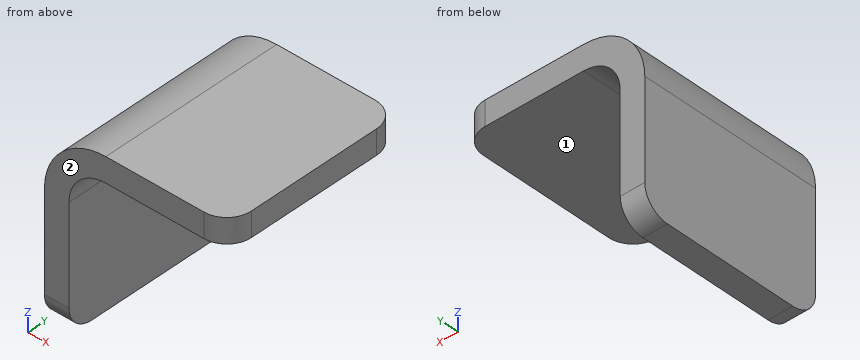
from build123d import *

# Parameters (mm, degrees)
F1_DEPTH = 15
F2_R     = 3
F3_R     = 5
F4_R     = 2


with BuildPart() as f1:
    # F0 (on Front) → F1 (new body)
    with BuildSketch(Plane.XZ):
        Polygon((15, 0), (0, 0), (0, -15), (2, -15), (2, -2), (15, -2), align=None)
    extrude(amount=F1_DEPTH)

    # F2
    f2_edges = [f1.edges().sort_by_distance(p)[0] for p in [
        (2, -7.5, -2),
    ]]
    fillet(f2_edges, radius=F2_R)

    # F3
    f3_edges = [f1.edges().sort_by_distance(p)[0] for p in [
        (0, -7.5, 0),
    ]]
    fillet(f3_edges, radius=F3_R)

    # F4
    f4_edges = [f1.edges().sort_by_distance(p)[0] for p in [
        (15, -15, -1),
        (15, 0, -1),
        (1, -15, -15),
        (1, 0, -15),
    ]]
    fillet(f4_edges, radius=F4_R)


solid = f1.part
For this review, take the finished solid that the model builds, in its own axes (mm). Face numbers are marked on the shaded views. A direction names the side the tool comes from. Round coordinates to 2 decimals unless told otherwise and drop trailing zeros. Order: outer loops, then holes, each group sorted by start corner. A loop starts at its lowest first (then second) coordinate and runs counter-clockwise, first axis right, second up. Notation, with made-up numbers: (6.5, -38) -> (10.5, -38) arc R24 ccw to (10.5, -14) -> close; hole circle Ø3 at (-5.5, -27.5). An arc over 180 degrees is marked (long way). Put each result on its own line as item: value.
Q1. Machinability: for the marked faces 1 and 2, which of the approach directions +Z, -Z, +X, -X, +Y, -Y give a long, thin tool a straight path to every point of the face, cutting with its end or side? Answer none if there is none.
Check result:
face 1: -Z, +X, +Y, -Y
face 2: +Z, -Z, +X, -X, -Y
Q2. Add section C-C on x = 11.5. Write out the cut boundary in (y, z).
Check result:
outline: (-15, -2) -> (0, -2) -> (0, 0) -> (-15, 0) -> close
Q3. For probe 1 along X at (y, z) = (-9.5, -12.75); probe 2 along Z at (x, y) = (8.5, -7.25); probe 3 along Z at (x, y) = (1, -8.75), list the stretches that pass through material, from the lowest coordinate up. Write a range as [from, to].
Check result:
probe 1: [0, 2]
probe 2: [-2, 0]
probe 3: [-15, -2]
Q4. Add section D-D on z = -1. Write out the cut boundary in (x, y).
Check result:
outline: (2, -15) -> (13, -15) arc R2 ccw to (15, -13) -> (15, -2) arc R2 ccw to (13, 0) -> (2, 0) -> close
Q5. Add section A-A on y = -12.5. Write out the cut boundary in (x, z).
Check result:
outline: (0, -15) -> (2, -15) -> (2, -5) arc R3 cw to (5, -2) -> (15, -2) -> (15, 0) -> (5, 0) arc R5 ccw to (0, -5) -> close
Q6. Add section B-B on z = -6. Write out the cut boundary in (x, y).
Check result:
outline: (0, -15) -> (2, -15) -> (2, 0) -> (0, 0) -> close
Q7. Insertion check: pin 1 Ø5 at (x, y) = (11, -5) entering from -Z; pin 2 Ø5 at (y, z) = (-5.5, -8.5) entering from +X. Each pin has a flat end and moves straight along its axis. Give the tip position at first contact, or say it passes through.
Check result:
pin 1: z = -2
pin 2: x = 2
